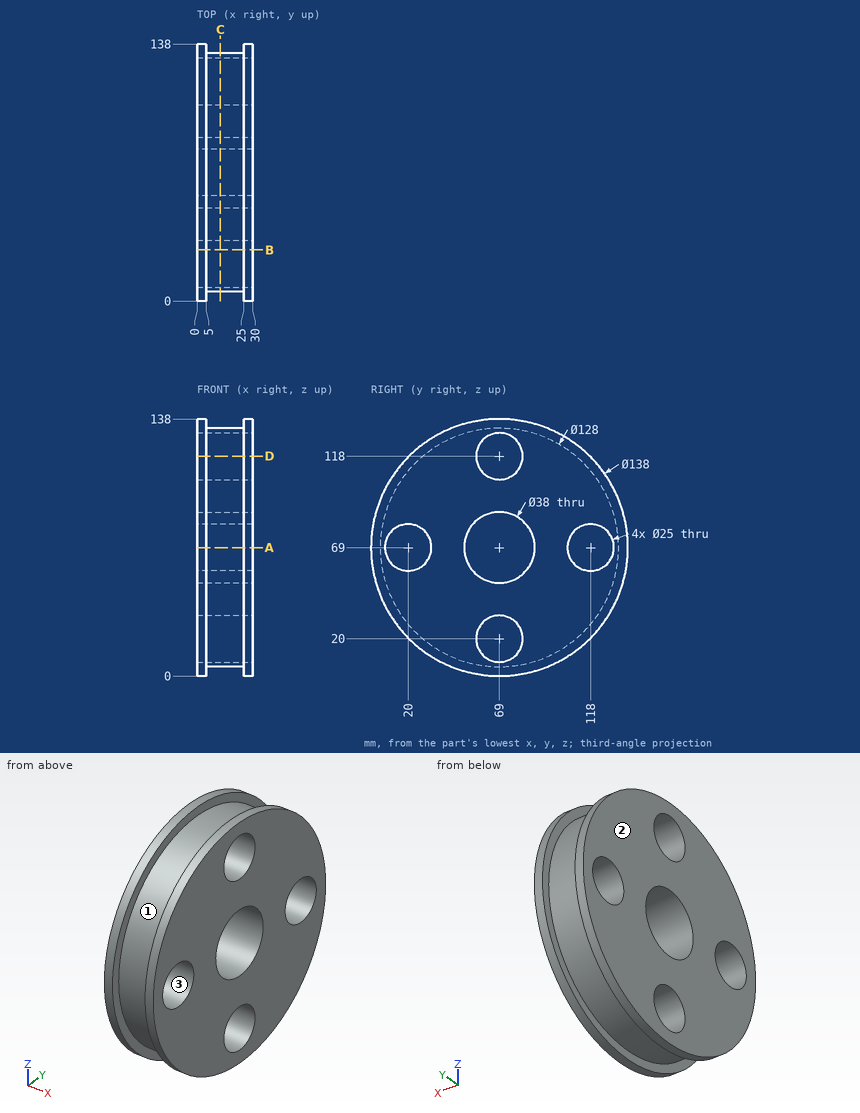
Print and shaded views of the part. All mm, measured from the part's lowest x, y and z. Round coordinates to 2 decimals unless told otherwise and drop trailing zeros. Loops run counter-clockwise (first coordinate to the right, second up) from the corner with the lowest first, then second, coordinate; pieces in that order, holes last. Notation, with made-up numbers: (89.5, 66.5) -> (129.5, 66.5) arc R22 cw to (129.5, 99.5) -> close; hole circle Ø5 at (-5.5, 52). An arc over 180 degrees is marked (long way). Use CSV: the item, a comma, the result in double quotes. Start each with the question number.
1) Cut at D-D, the plane z = 118. Write the cut outline in (x, y), plus the area to 3 significant figures.
2) Drop flat-ended pins along their axis: P1, Ø8, axis at y = 38, z = 15.5, coming from the -X side; P2, Ø1.5, axis at x = 15, z = 67, coming from the +Y side; P3, Ø3, axis at x = 22, y = 15, coming from the +Z side; P4, Ø12, axis at x = 3.5, z = 28.5, coming from the +Y side. Give the stop position or say it passes through.
3) Cut at B-B, the plane y = 27.5. Write the cut outline in (x, z), plus the area to 3 significant figures.
4) Wall check: L1, parallel to Z at x = 17.5, y = 69; L2, parallel to X at y = 31.5, z = 15.5. Give the ranges that are in metal, low to high. Write a range as [from, to].
5) Cut at A-A, the plane z = 69. Write the cut outline in (x, y).
6) Pull direction Z, two halves, no side cores. Call the marked faces 1, 2 and 3: +Z half, -Z half, draft (parallel to the pull), parting line (faces both ways), or undercut.
7) Cut at C-C, the plane x = 12.5. Write the cut outline in (y, z), plus the area to 3 significant figures.
Determined:
1,outline,"(0, 20.42) -> (5, 20.42) -> (5, 27.83) -> (25, 27.83) -> (25, 20.42) -> (30, 20.42) -> (30, 56.5) -> (0, 56.5) -> close; (0, 81.5) -> (30, 81.5) -> (30, 117.58) -> (25, 117.58) -> (25, 110.17) -> (5, 110.17) -> (5, 117.58) -> (0, 117.58) -> close"
1,area,"1,870 mm2"
2,P1,"stops at x = 0"
2,P2,"stops at y = 132.99"
2,P3,"stops at z = 105.6"
2,P4,"stops at y = 128.76"
3,outline,"(0, 13.88) -> (5, 13.88) -> (5, 20.28) -> (25, 20.28) -> (25, 13.88) -> (30, 13.88) -> (30, 59) -> (0, 59) -> close; (0, 79) -> (30, 79) -> (30, 124.12) -> (25, 124.12) -> (25, 117.72) -> (5, 117.72) -> (5, 124.12) -> (0, 124.12) -> close"
3,area,"2,450 mm2"
4,L1,"z = [5, 7.5], [32.5, 50], [88, 105.5], [130.5, 133]"
4,L2,"x = [0, 5], [25, 30]"
5,outline,"(0, 0) -> (5, 0) -> (5, 5) -> (25, 5) -> (25, 0) -> (30, 0) -> (30, 7.5) -> (0, 7.5) -> close; (0, 32.5) -> (30, 32.5) -> (30, 50) -> (0, 50) -> close; (0, 88) -> (30, 88) -> (30, 105.5) -> (0, 105.5) -> close; (0, 130.5) -> (30, 130.5) -> (30, 138) -> (25, 138) -> (25, 133) -> (5, 133) -> (5, 138) -> (0, 138) -> close"
6,face 1,"parting line"
6,face 2,"draft"
6,face 3,"undercut"
7,outline,"circle Ø128 at (69, 69); hole circle Ø25 at (20, 69); hole circle Ø38 at (69, 69); hole circle Ø25 at (69, 20); hole circle Ø25 at (69, 118); hole circle Ø25 at (118, 69)"
7,area,"9,770 mm2"
